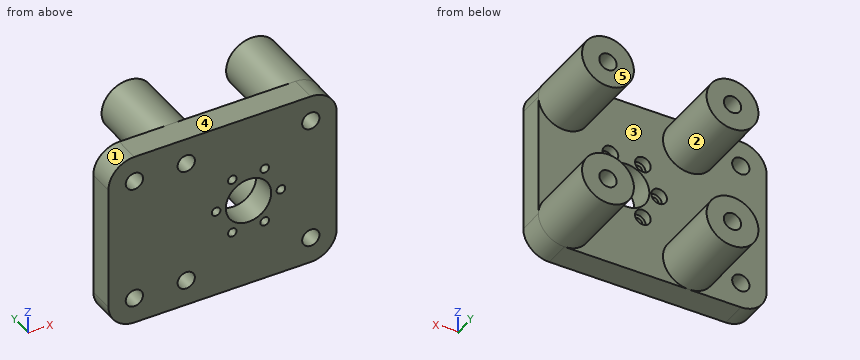
from build123d import *

# Parameters (mm, degrees)
SKETCH1_R                = 4
SKETCH1_R_2              = 10.5
SKETCH1_R_3              = 2
BASE_DEPTH               = 12
SKETCH2_R                = 3.625
BOLT_HEAD_RECESSES_DEPTH = 4
SKETCH3_R                = 12
SKETCH3_R_2              = 4
BOSS_EXTRUDE1_DEPTH      = 34.5


with BuildPart() as part:
    # Sketch1 → base (new body)
    with BuildSketch(Plane(origin=(0, 0, 0), x_dir=(1, 0, 0), z_dir=(0, 1, 0))):
        with BuildLine():
            Line((-52.814601333, 40.814601333), (28.814601333, 40.814601333))
            ThreePointArc((28.814601333, 40.814601333), (37.299882708, 37.299882708), (40.814601333, 28.814601333))
            Line((40.814601333, 28.814601333), (40.814601333, -28.814601333))
            ThreePointArc((40.814601333, -28.814601333), (37.299882708, -37.299882708), (28.814601333, -40.814601333))
            Line((28.814601333, -40.814601333), (-52.814601333, -40.814601333))
            ThreePointArc((-52.814601333, -40.814601333), (-61.299882708, -37.299882708), (-64.814601333, -28.814601333))
            Line((-64.814601333, -28.814601333), (-64.814601333, 28.814601333))
            ThreePointArc((-64.814601333, 28.814601333), (-61.299882708, 37.299882708), (-52.814601333, 40.814601333))
        make_face()
        with Locations(Location((-28.814601333, 28.814601333, 0), (0, 0, 270))):
            Circle(SKETCH1_R, mode=Mode.SUBTRACT)
        with Locations(Location((28.814601333, 28.814601333, 0), (0, 0, 270))):
            Circle(SKETCH1_R, mode=Mode.SUBTRACT)
        with Locations(Location((28.814601333, -28.814601333, 0), (0, 0, 270))):
            Circle(SKETCH1_R, mode=Mode.SUBTRACT)
        with Locations(Location((-28.814601333, -28.814601333, 0), (0, 0, 270))):
            Circle(SKETCH1_R, mode=Mode.SUBTRACT)
        with Locations(Location((0, 0, 0), (0, 0, 270))):
            Circle(SKETCH1_R_2, mode=Mode.SUBTRACT)
        with Locations(Location((-7.5, 12.990381057, 0), (0, 0, 270))):
            Circle(SKETCH1_R_3, mode=Mode.SUBTRACT)
        with Locations(Location((7.5, 12.990381057, 0), (0, 0, 270))):
            Circle(SKETCH1_R_3, mode=Mode.SUBTRACT)
        with Locations(Location((15, 0, 0), (0, 0, 270))):
            Circle(SKETCH1_R_3, mode=Mode.SUBTRACT)
        with Locations(Location((7.5, -12.990381057, 0), (0, 0, 270))):
            Circle(SKETCH1_R_3, mode=Mode.SUBTRACT)
        with Locations(Location((-7.5, -12.990381057, 0), (0, 0, 270))):
            Circle(SKETCH1_R_3, mode=Mode.SUBTRACT)
        with Locations(Location((-15, 0, 0), (0, 0, 270))):
            Circle(SKETCH1_R_3, mode=Mode.SUBTRACT)
        with Locations(Location((-52.814601333, 28.814601333, 0), (0, 0, 270))):
            Circle(SKETCH1_R, mode=Mode.SUBTRACT)
        with Locations(Location((-52.814601333, -28.814601333, 0), (0, 0, 270))):
            Circle(SKETCH1_R, mode=Mode.SUBTRACT)
    extrude(amount=BASE_DEPTH)

    # Sketch2 → bolt head recesses (cut)
    with BuildSketch(Plane(origin=(0, 12, 0), x_dir=(1, 0, 0), z_dir=(0, 1, 0))):
        with Locations(Location((-7.5, 12.990381057, 0), (0, 0, 270))):
            Circle(SKETCH2_R)
        with Locations(Location((7.5, 12.990381057, 0), (0, 0, 270))):
            Circle(SKETCH2_R)
        with Locations(Location((15, 0, 0), (0, 0, 270))):
            Circle(SKETCH2_R)
        with Locations(Location((7.5, -12.990381057, 0), (0, 0, 270))):
            Circle(SKETCH2_R)
        with Locations(Location((-7.5, -12.990381057, 0), (0, 0, 270))):
            Circle(SKETCH2_R)
        with Locations(Location((-15, 0, 0), (0, 0, 270))):
            Circle(SKETCH2_R)
    extrude(amount=-BOLT_HEAD_RECESSES_DEPTH, mode=Mode.SUBTRACT)

    # Sketch3 → Boss-Extrude1 (add)
    # profile 1 of 4: a face of its own
    with BuildSketch(Plane(origin=(0, 12, 0), x_dir=(1, 0, 0), z_dir=(0, 1, 0))):
        with Locations(Location((-28.814601333, 28.814601333, 0), (0, 0, 90))):
            Circle(SKETCH3_R)
        with Locations(Location((-28.814601333, 28.814601333, 0), (0, 0, 270))):
            Circle(SKETCH3_R_2, mode=Mode.SUBTRACT)
    # profile 2 of 4: a face of its own
    with BuildSketch(Plane(origin=(0, 12, 0), x_dir=(1, 0, 0), z_dir=(0, 1, 0))):
        with Locations(Location((28.814601333, 28.814601333, 0), (0, 0, 90))):
            Circle(SKETCH3_R)
        with Locations(Location((28.814601333, 28.814601333, 0), (0, 0, 270))):
            Circle(SKETCH3_R_2, mode=Mode.SUBTRACT)
    # profile 3 of 4: a face of its own
    with BuildSketch(Plane(origin=(0, 12, 0), x_dir=(1, 0, 0), z_dir=(0, 1, 0))):
        with Locations(Location((28.814601333, -28.814601333, 0), (0, 0, 270))):
            Circle(SKETCH3_R)
        with Locations(Location((28.814601333, -28.814601333, 0), (0, 0, 270))):
            Circle(SKETCH3_R_2, mode=Mode.SUBTRACT)
    # profile 4 of 4: a face of its own
    with BuildSketch(Plane(origin=(0, 12, 0), x_dir=(1, 0, 0), z_dir=(0, 1, 0))):
        with Locations(Location((-28.814601333, -28.814601333, 0), (0, 0, 270))):
            Circle(SKETCH3_R)
        with Locations(Location((-28.814601333, -28.814601333, 0), (0, 0, 270))):
            Circle(SKETCH3_R_2, mode=Mode.SUBTRACT)
    extrude(amount=BOSS_EXTRUDE1_DEPTH)


solid = part.part
Could you check a few things on this model? Use its own coordinates, in mm. Face numbers are marked on the shaded views. A direction names the side the tool comes from. Round coordinates to 2 decimals unless told otherwise and drop trailing zeros. Order: outer loops, then holes, each group sorted by start corner. A loop starts at its lowest first (then second) coordinate and runs counter-clockwise, first axis right, second up.
Q1. Imagine slicing it at A-A, the plane x = 0. List the corners of the cut face in (y, z) for me.
Geometry says:
outline: (0, -40.81) - (12, -40.81) - (12, -10.5) - (0, -10.5) - close; (0, 10.5) - (12, 10.5) - (12, 40.81) - (0, 40.81) - close
Q2. Imagine slicing it at B-B, the plane z = 0. List the corners of the cut face in (x, y) for me (3 decimals), then the cut area to 3 significant figures.
Geometry says:
outline: (-64.815, 0) - (-17, 0) - (-17, 8) - (-18.625, 8) - (-18.625, 12) - (-64.815, 12) - close; (-13, 0) - (-10.5, 0) - (-10.5, 12) - (-11.375, 12) - (-11.375, 8) - (-13, 8) - close; (10.5, 0) - (13, 0) - (13, 8) - (11.375, 8) - (11.375, 12) - (10.5, 12) - close; (17, 0) - (40.815, 0) - (40.815, 12) - (18.625, 12) - (18.625, 8) - (17, 8) - close
area: 894 mm2
Q3. Please list where these lines run through material, in increasing order: probe 1 along X at (y, z) = (2, 0); probe 2 along X at (y, z) = (19, -29); probe 3 along Z at (x, y) = (-52, 10).
Geometry says:
probe 1: x = -64.81 to -17, -13 to -10.5, 10.5 to 13, 17 to 40.81
probe 2: x = -40.81 to -32.81, -24.82 to -16.82, 16.82 to 24.82, 32.81 to 40.81
probe 3: z = -40.81 to -32.73, -24.9 to 24.9, 32.73 to 40.81
Q4. Imagine slicing it at C-C, the plane y = 40. List the corners of the cut face in (x, z) for me, then the cut area to 3 significant figures.
Geometry says:
outline: circle Ø24 at (-28.81, -28.81); circle Ø24 at (-28.81, 28.81); circle Ø24 at (28.81, -28.81); circle Ø24 at (28.81, 28.81); hole circle Ø8 at (-28.81, -28.81); hole circle Ø8 at (-28.81, 28.81); hole circle Ø8 at (28.81, -28.81); hole circle Ø8 at (28.81, 28.81)
area: 1,610 mm2
Q5. I'm going to push flat-ended pins straight in: P1, Ø12, axis at y = 38.5, z = -27, coming from the -X side; P2, Ø6, axis at y = 16, z = 13, coming from the -X side; P3, Ø6, axis at x = -7.5, z = 12.99, coming from the +Y side; P4, Ø8, axis at x = 7, z = 14, coming from the +Y side. Where does each tip first touch, or does it pass through?
Geometry says:
P1: stops at x = -40.81
P2: passes through
P3: stops at y = 8
P4: stops at y = 12
Q6. Thinking about a two-plate mould opening in Z: for the marked faces 3, 4 and 5, which applies, released by +Z, released by -Z, zero draft, split by the parting line, or undercut?
Geometry says:
face 3: undercut
face 4: released by +Z
face 5: zero draft
Q7. Which directions (+Z, -Z, +X, -X, +Y, -Y) give clear straight access to the entire face, cutting with the end or side of a thin tool? Please do the marked faces 1 and 2.
Geometry says:
face 1: +Z, -X, +Y, -Y
face 2: +Y
Q8. Imagine slicing it at D-D, the plane x = 31. List the corners of the cut face in (y, z) for me.
Geometry says:
outline: (0, -40.61) - (46.5, -40.61) - (46.5, -32.16) - (0, -32.16) - close; (0, -25.46) - (46.5, -25.46) - (46.5, -17.02) - (12, -17.02) - (12, 17.02) - (46.5, 17.02) - (46.5, 25.46) - (0, 25.46) - close; (0, 32.16) - (46.5, 32.16) - (46.5, 40.61) - (0, 40.61) - close
